Autodesk Fusion 360 part; units mm, degrees
sketch "Sketch1" plane through (0, 0, 0) normal (0, 0, 1) x (1, 0, 0)
  circle A0 centre (0, 0) radius 55
  circle A1 centre (0, 0) radius 4
  circle A2 centre (0, 0) radius 3.15
  dimension "d1" = 110
  dimension "d2" = 8
  dimension "d3" = 6.3
extrude "Extrude1" add sketch "Sketch1" against normal blind 1 contours A0
extrude "Extrude2" add sketch "Sketch1" against normal blind 1 contours A1
extrude "Extrude3" add sketch "Sketch1" along normal blind 180 contours A1
equation "d3 = 8 mm - 1.7 mm"
Here's how the part is built. I have some questions about the finished solid (model axes, mm). Coordinates: 2 decimals unless noted, no trailing zeros. Loops run counter-clockwise (first coordinate to the right, second up) from the corner with the lowest first, then second, coordinate; pieces in that order, holes last.
1. I need wall thicknesses on L1, parallel to Y at x = 0, z = 101; L2, parallel to Z at x = 32, y = 36.5; L3, parallel to X at y = -1, z = 142. Which ranges of each line are inside material? Lowest first, please.
2. Imagine slicing it at D-D, the plane x = 47.5. Please give me the cut outline in (y, z).
3. For P1, Ø1, axis at y = 2, z = 92.5, coming from the +X side; P2, Ø6, axis at y = -5.5, z = 132.5, coming from the -X side, each with a flat end and sliding along its axis, tell me the tip position at first contact or that it passes through.
4. Imagine slicing it at C-C, the plane z = 88.5. Please give me the cut outline in (x, y).
5. If we mould it in two halves opening along X, with no side actions, what happens to faces 1 (the flat face through (2, -3, 180)), 2 (the cylindrical face through (-2.5, 1.917, 88.233)), 3 (the cylindrical face through (-0.867, 3.905, 88.74))? For each: pulls with the +X half, pulls with the -X half, needs draft (parallel to the pull), parting line crosses it, or undercut.
6. Imagine slicing it at A-A, the plane y = 0. Please give me the cut outline in (x, z), and give its area (3 significant figures).
Taken from the geometry:
1. L1: y = -4 to -3.15, 3.15 to 4
1. L2: z = -1 to 0
1. L3: x = -3.87 to -2.99, 2.99 to 3.87
2. outline: (-27.73, -1) - (27.73, -1) - (27.73, 0) - (-27.73, 0) - close
3. P1: stops at x = 3.71
3. P2: stops at x = -3.12
4. outline: circle Ø8 at (0, 0); hole circle Ø6.3 at (0, 0)
5. face 1: needs draft
5. face 2: undercut
5. face 3: parting line crosses it
6. outline: (-55, -1) - (-3.15, -1) - (-3.15, 180) - (-4, 180) - (-4, 0) - (-55, 0) - close; (3.15, -1) - (55, -1) - (55, 0) - (4, 0) - (4, 180) - (3.15, 180) - close
6. area: 410 mm2
